Autodesk Inventor part; units mm, degrees
ref_plane "YZ Plane" through (0, 0, 0) normal (1, 0, 0) x (0, 1, 0)
ref_plane "XZ Plane" through (0, 0, 0) normal (0, 1, 0) x (-1, 0, 0)
ref_plane "XY Plane" through (0, 0, 0) normal (0, 0, 1) x (1, 0, 0)
sketch "Skizze1" plane through (0, 0, 0) normal (0, 0, 1) x (1, 0, 0)
  line L0 (-41.25, -314) -> (-33.75, -314)
  line L1 (-41.25, -312) -> (-41.25, -314)
  line L2 (-11.25, -312) -> (-41.25, -312)
  line L3 (-18.75, -314) -> (-11.25, -314)
  line L4 (-11.25, -314) -> (-11.25, -312)
  line L5 (-18.75, -314) -> (-16.75, -314)
  line L6 (-16.75, -314) -> (-16.75, -321)
  line L7 (-16.75, -321) -> (-4.75, -321)
  line L8 (-4.75, -321) -> (-4.75, -305)
  line L9 (-4.75, -305) -> (-70.75, -305)
  line L10 (-70.75, -305) -> (-70.75, -314)
  line L11 (-47.75, -314) -> (-47.75, -321)
  line L12 (-47.75, -321) -> (-35.75, -321)
  line L13 (-35.75, -321) -> (-35.75, -314)
  line L14 (-35.75, -314) -> (-33.75, -314)
  line L15 (-70.75, -314) -> (-65.75, -314)
  line L16 (-65.75, -314) -> (-65.75, -315)
  line L17 (-65.75, -315) -> (-62.75, -315)
  line L18 (-62.75, -315) -> (-62.75, -314)
  line L19 (-62.75, -314) -> (-47.75, -314)
  line L20 (-23.75, -312) -> (-23.75, -311)
  line L21 (-23.75, -311) -> (-26.25, -311)
  line L22 (-26.25, -311) -> (-28.75, -311)
  line L23 (-28.75, -311) -> (-28.75, -312)
  line L24 (-26.25, -311) -> (-26.25, -312) construction
  point P0 (0, 0)
  point P1 (-64.25, -315)
  dimension "d0" = 2
  dimension "d1" = 7
  dimension "d2" = 12
  dimension "d3" = 16
  dimension "d4" = 12
  dimension "d5" = 2
  dimension "d6" = 3
  dimension "d7" = 38
  dimension "d8" = 5
  dimension "d9" = 1
  dimension "d20" = 1
  dimension "d21" = 5
extrude "Extrusion1" add sketch "Skizze1" along normal blind 30 contours L0 L13 L12 L11 L19 L18 L17 L16 L15 L10 L9 L8 L7 L6 L3 L4 L2 L20 L21 L22 L23 L1
chamfer "Fasen1" distance 1 distance2 13.5 1 edges at (-64.25, -315, 30) measured on face at (-34.75, -307, 30)
chamfer "Fasen2" distance 1 distance2 13.5 1 edges at (-64.25, -315, 0) measured on face at (-34.75, -307, 0)
sketch "Skizze2" plane through (-70.75, -305, 0) normal (0, 1, 0) x (1, 0, 0)
  line L0 (29.5, 0) -> (59.5, 0)
  line L1 (59.5, 0) -> (59.5, -30)
  line L2 (29.5, 0) -> (59.5, 0)
  line L3 (59.5, 0) -> (59.5, -30)
  line L4 (59.5, -30) -> (29.5, -30)
  line L5 (29.5, -30) -> (29.5, 0)
  point P0 (70.75, 0)
extrude "Extrusion2" add sketch "Skizze2" along normal blind 1
properties part number "KatzeFEM" material "Aluminium 6061, Katze"
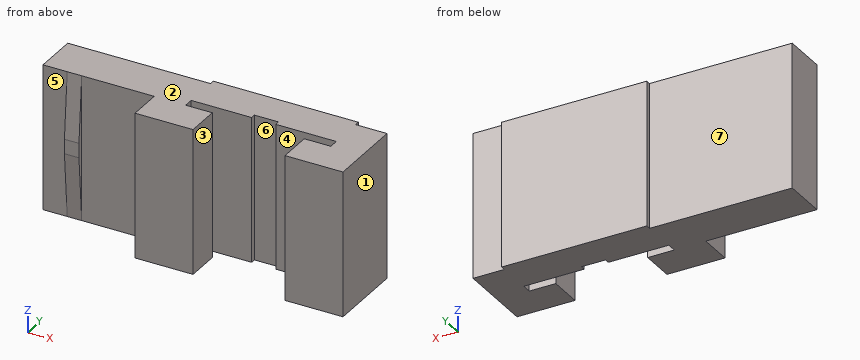
For this review, take the finished solid that the model builds, in its own axes (mm). Face numbers are marked on the shaded views. A direction names the side the tool comes from. Give positions to 0.01 mm unless a question says otherwise; leave off trailing zeros. Order: outer loops, then holes, each group sorted by start corner. A loop starts at its lowest first (then second) coordinate and runs counter-clockwise, first axis right, second up. Notation, with made-up numbers: (43.5, 74) - (55.5, 74) arc R15 ccw to (55.5, 78) - close; hole circle Ø8 at (-4, -16). An arc over 180 degrees is marked (long way). Answer as a JSON object with one key per item and string values. Group by question number.
Item 1: Draft analysis for pull direction X (two halves, no side actions). For the marked faces 1, 2 and 3, state which applies: pulls with the +X half, pulls with the -X half, needs draft (parallel to the pull), parting line crosses it, or undercut.
Item 2: Take a section at A-A on y = -313. Give the boundary of the cut face in (x, z).
Item 3: Take a section at D-D on x = -32.5. Give the boundary of the cut face in (y, z), and give its area (3 significant figures).
Item 4: Clearance check with flat-ended pins moving along their axes: pin 1 Ø1 at (x, y) = (-54.5, -315) entering from -Z; pin 2 Ø7 at (x, z) = (-9, 20) entering from +Y; pin 3 Ø5 at (x, z) = (-59.5, 6) entering from +Y; pin 4 Ø5.5 at (x, z) = (-26.5, 22.5) entering from -Y. State where each tip first meets the part, or that it passes through.
Item 5: Take a section at C-C on z = 22. Give the boundary of the cut face in (x, y), and give its area (3 significant figures).
Item 6: Machinability: for the marked faces 4, 5, 6 and 7, which of the approach directions +Z, -Z, +X, -X, +Y, -Y give a long, thin tool a straight path to every point of the face, cutting with its end or side? Answer none if there is none.
Item 7: Wall thickness on line 1 along X through (y, z) = (-317, 7); line 2 along Y through (x, z) = (-38.5, 16); line 3 along X through (y, z) = (-312.25, 12): over which ranges is each line inside the solid? List them lowest first.
Item 8: Take a section at B-B on x = -15.5. Give the boundary of the cut face in (y, z), and give its area (3 significant figures).
Reported:
{
 "1": {"face 1": "pulls with the +X half", "face 2": "needs draft", "face 3": "undercut"},
 "2": {"outline": "(-70.75, 0) - (-41.25, 0) - (-41.25, 30) - (-70.75, 30) - close; (-11.25, 0) - (-4.75, 0) - (-4.75, 30) - (-11.25, 30) - close"},
 "3": {"outline": "(-312, 0) - (-304, 0) - (-304, 30) - (-312, 30) - close", "area": "240 mm^2"},
 "4": {"pin 1": "through", "pin 2": "y = -304", "pin 3": "y = -305", "pin 4": "y = -312"},
 "5": {"outline": "(-70.75, -314) - (-65.75, -314) - (-65.75, -314.59) - (-62.75, -314.59) - (-62.75, -314) - (-47.75, -314) - (-47.75, -321) - (-35.75, -321) - (-35.75, -314) - (-41.25, -314) - (-41.25, -312) - (-28.75, -312) - (-28.75, -311) - (-23.75, -311) - (-23.75, -312) - (-11.25, -312) - (-11.25, -314) - (-16.75, -314) - (-16.75, -321) - (-4.75, -321) - (-4.75, -305) - (-11.25, -305) - (-11.25, -304) - (-41.25, -304) - (-41.25, -305) - (-70.75, -305) - close", "area": "729 mm^2"},
 "6": {"face 4": "+Z, -Z", "face 5": "+Z, -Z, -X, -Y", "face 6": "+Z, -Z, -Y", "face 7": "+Z, -Z, -X, +Y"},
 "7": {"line 1": "-47.75 to -35.75, -16.75 to -4.75", "line 2": "-321 to -314, -312 to -304", "line 3": "-70.75 to -41.25, -11.25 to -4.75"},
 "8": {"outline": "(-321, 0) - (-314, 0) - (-314, 30) - (-321, 30) - close; (-312, 0) - (-304, 0) - (-304, 30) - (-312, 30) - close", "area": "450 mm^2"}
}
